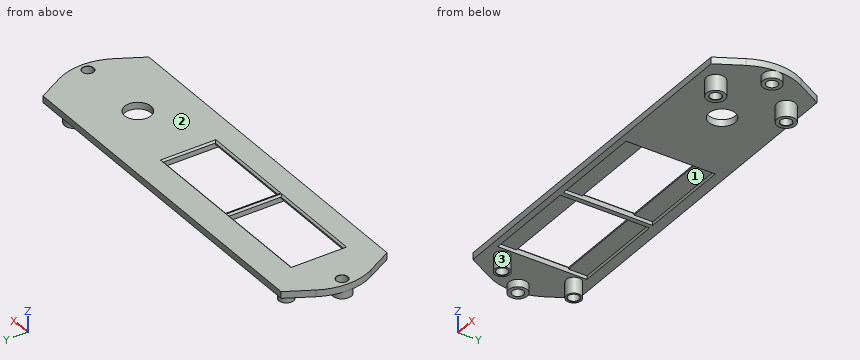
```python
from build123d import *

# Parameters (mm, degrees)
BOSS_EXTRUDE1_DEPTH             = 1.905
SKETCH6_R                       = 2.629225159
BOSS_EXTRUDE4_DEPTH             = 2.095
F_3_0MM_DOWEL_HOLE1_D           = 3.2
F_3_0MM_DOWEL_HOLE1_CSINK_D     = 3.3
F_3_0MM_DOWEL_HOLE1_CSINK_ANGLE = 90
SKETCH7_R                       = 3.75
SKETCH7_W                       = 26.6
SKETCH7_H                       = 14.7701
CUT_EXTRUDE1_DEPTH              = 59.70468385
SKETCH9_R                       = 2.629225159
SKETCH9_R_2                     = 2.125
BOSS_EXTRUDE5_DEPTH             = 4.5
F_3_0MM_DOWEL_HOLE2_D           = 3.1
F_3_0MM_DOWEL_HOLE2_DEPTH       = 4
F_3_0MM_DOWEL_HOLE2_CSINK_D     = 3.3
F_3_0MM_DOWEL_HOLE2_CSINK_ANGLE = 90
F_3_0MM_DOWEL_HOLE2_TIP         = 0.931333959
SKETCH12_W                      = 26.6
SKETCH12_H                      = 25.3701
CUT_EXTRUDE2_DEPTH              = 1
CHAMFER1_SIZE                   = 0.5


with BuildPart() as part:
    # Sketch1 → Boss-Extrude1 (new body)
    with BuildSketch(Plane.XY):
        with BuildLine():
            Line((-50.6, 15.04), (50.6, 15.04))
            Line((50.6, 15.04), (54.590317598, 7.813493896))
            ThreePointArc((54.590317598, 7.813493896), (56.604225159, 0), (54.590317598, -7.813493896))
            Line((54.590317598, -7.813493896), (50.6, -15.04))
            Line((50.6, -15.04), (-50.6, -15.04))
            Line((-50.6, -15.04), (-54.590317598, -7.813493896))
            ThreePointArc((-54.590317598, -7.813493896), (-56.604225159, 0), (-54.590317598, 7.813493896))
            Line((-54.590317598, 7.813493896), (-50.6, 15.04))
        make_face()
    extrude(amount=BOSS_EXTRUDE1_DEPTH)

    # Sketch6 → Boss-Extrude4 (add)
    with BuildSketch(Plane(origin=(0, 0, 0), x_dir=(-1, 0, 0), z_dir=(0, 0, -1))):
        with Locations(Location((-53.975, 0, 0), (0, 0, 179.99945392))):
            Circle(SKETCH6_R)
        with Locations(Location((53.975, 0, 0), (0, 0, 359.99945398))):
            Circle(SKETCH6_R)
    extrude(amount=BOSS_EXTRUDE4_DEPTH)

    # Ø3.0mm Dowel Hole1 (through all)
    with Locations(Plane.XY.offset(1.905)):
        with Locations((53.975, 0), (-53.975, 0)):
            CounterSinkHole(F_3_0MM_DOWEL_HOLE1_D / 2, F_3_0MM_DOWEL_HOLE1_CSINK_D / 2, counter_sink_angle=F_3_0MM_DOWEL_HOLE1_CSINK_ANGLE)

    # Sketch7 → Cut-Extrude1 (cut, through all)
    with BuildSketch(Plane.XY.offset(1.905)):
        with Locations((32.762, 0)):
            Circle(SKETCH7_R)
        with Locations((-29.464, -0.57505)):
            Rectangle(SKETCH7_W, SKETCH7_H)
        with Locations((-1.524, -0.57505)):
            Rectangle(SKETCH7_W, SKETCH7_H)
    extrude(amount=-CUT_EXTRUDE1_DEPTH, mode=Mode.SUBTRACT)

    # Sketch9 → Boss-Extrude5 (add)
    with BuildSketch(Plane(origin=(0, 0, 0), x_dir=(-1, 0, 0), z_dir=(0, 0, -1))):
        with Locations((-45.212, 9.906)):
            Circle(SKETCH9_R)
        with Locations((-45.212, -10.16)):
            Circle(SKETCH9_R)
        with Locations((45.466, -10.16)):
            Circle(SKETCH9_R_2)
        with Locations((45.466, 10.16)):
            Circle(SKETCH9_R_2)
    extrude(amount=BOSS_EXTRUDE5_DEPTH)

    # Ø3.0mm Dowel Hole2
    with Locations(Plane(origin=(0, 0, -4.5), x_dir=(-1, 0, 0), z_dir=(0, 0, -1))):
        with Locations((-45.212, 9.906), (-45.212, -10.16), (45.466, -10.16), (45.466, 10.16)):
            CounterSinkHole(F_3_0MM_DOWEL_HOLE2_D / 2, F_3_0MM_DOWEL_HOLE2_CSINK_D / 2, depth=F_3_0MM_DOWEL_HOLE2_DEPTH, counter_sink_angle=F_3_0MM_DOWEL_HOLE2_CSINK_ANGLE)
            with Locations((0, 0, -(F_3_0MM_DOWEL_HOLE2_DEPTH + F_3_0MM_DOWEL_HOLE2_TIP / 2))):  # 118° drill point
                Cone(0, F_3_0MM_DOWEL_HOLE2_D / 2, F_3_0MM_DOWEL_HOLE2_TIP, mode=Mode.SUBTRACT)

    # Sketch12 → Cut-Extrude2 (cut)
    with BuildSketch(Plane(origin=(0, 0, 0), x_dir=(-1, 0, 0), z_dir=(0, 0, -1))):
        with Locations((1.524, -0.57505)):
            Rectangle(SKETCH12_W, SKETCH12_H)
        with Locations((29.464, -0.57505)):
            Rectangle(SKETCH12_W, SKETCH12_H)
    extrude(amount=-CUT_EXTRUDE2_DEPTH, mode=Mode.SUBTRACT)

    # Chamfer1
    chamfer1_edges = [part.edges().sort_by_distance(p)[0] for p in [
        (-42.764, -0.57505, 1.905),
        (-29.464, -7.9601, 1.905),
        (-16.164, -0.57505, 1.905),
        (-29.464, 6.81, 1.905),
        (-14.824, -0.57505, 1.905),
        (-1.524, -7.9601, 1.905),
        (11.776, -0.57505, 1.905),
        (-1.524, 6.81, 1.905),
    ]]
    chamfer(chamfer1_edges, length=CHAMFER1_SIZE)


solid = part.part
```
Verification items for the finished model (mm, model axes). Face numbers are marked on the shaded views. Coordinates: 2 decimals unless noted, no trailing zeros. Loops run counter-clockwise (first coordinate to the right, second up) from the corner with the lowest first, then second, coordinate; pieces in that order, holes last. Notation, with made-up numbers: (-23, 46) -> (20, 46) arc R21 ccw to (20, 68) -> close; hole circle Ø1 at (79, 77.5). An arc over 180 degrees is marked (long way). Put each result on its own line as item: value.
1. Mould release check, pull along Y, two halves, no side actions. Record for the marked faces 1, 2 and 3: pulls with the +Y half, pulls with the -Y half, needs draft (parallel to the pull), parting line crosses it, or undercut.
Result set:
face 1: undercut
face 2: needs draft
face 3: undercut
2. Gauge pin test, flat ends, axial feed: P1, Ø12, axis at x = 7.5, y = 0.5, coming from the +Z side (3 decimals); P2, Ø12, axis at x = 32.762, y = 0, coming from the -Z side; P3, Ø3, axis at x = 45.212, y = -10.16, coming from the -Z side; P4, Ø2.5, axis at x = -7.5, y = -9.5, coming from the -Z side. Record the tip position at first contact, or that the pin passes through.
Result set:
P1: stops at z = 1.905
P2: stops at z = 0
P3: stops at z = -0.47
P4: stops at z = 1
3. Thickness scan on line 1 (X direction, y = 0, z = -0.85) (3 decimals); line 2 (X direction, y = -10.5, z = 0.75); line 3 (X direction, y = -6.5, z = 0.25). Record the ranges inside material, lowest first.
Result set:
line 1: x = -56.604 to -55.575, -52.375 to -51.346, 51.346 to 52.375, 55.575 to 56.604
line 2: x = -53.11 to -42.76, -16.16 to -14.82, 11.78 to 53.11
line 3: x = -55.24 to -42.76, -16.16 to -14.82, 11.78 to 55.24
4. Section check A-A, the plane x = 9. Record the boundary of the cut face in (y, z) (3 decimals).
Result set:
outline: (-15.04, 0) -> (-13.26, 0) -> (-13.26, 1) -> (-7.96, 1) -> (-7.96, 1.405) -> (-8.46, 1.905) -> (-15.04, 1.905) -> close; (6.81, 1) -> (12.11, 1) -> (12.11, 0) -> (15.04, 0) -> (15.04, 1.905) -> (7.31, 1.905) -> (6.81, 1.405) -> close
5. Section check B-B, the plane y = -5. Record the boundary of the cut face in (x, z) (3 decimals), then the cut area to 3 significant figures.
Result set:
outline: (-55.811, 0) -> (-42.764, 0) -> (-42.764, 1.405) -> (-43.264, 1.905) -> (-55.811, 1.905) -> close; (-16.164, 0) -> (-14.824, 0) -> (-14.824, 1.405) -> (-15.324, 1.905) -> (-15.664, 1.905) -> (-16.164, 1.405) -> close; (11.776, 0) -> (55.811, 0) -> (55.811, 1.905) -> (12.276, 1.905) -> (11.776, 1.405) -> close
area: 111 mm^2
